```python
from build123d import *

# Parameters (mm, degrees)
F0_W     = 31.6992
F0_H     = 15.9004
F0_R     = 2.3876
F1_DEPTH = 3.175
F2_DEPTH = 4.7752
F3_T     = -1.6002


with BuildPart() as f1:
    # F0 (on Top) → F1 (new body)
    with BuildSketch(Plane.XY):
        with Locations((0.5139857531, -7.2151332219)):
            Rectangle(F0_W, F0_H)
        with Locations((-11.3732142469, -11.1521332219)):
            Circle(F0_R, mode=Mode.SUBTRACT)
        with Locations((-3.4230142469, -11.1521332219)):
            Circle(F0_R, mode=Mode.SUBTRACT)
        with Locations((4.5271857531, -11.1521332219)):
            Circle(F0_R, mode=Mode.SUBTRACT)
        with Locations((12.4773857531, -11.1521332219)):
            Circle(F0_R, mode=Mode.SUBTRACT)
        with Locations((-11.3732142469, -3.2273332219)):
            Circle(F0_R, mode=Mode.SUBTRACT)
        with Locations((-3.4230142469, -3.2273332219)):
            Circle(F0_R, mode=Mode.SUBTRACT)
        with Locations((4.5271857531, -3.2273332219)):
            Circle(F0_R, mode=Mode.SUBTRACT)
        with Locations((12.4773857531, -3.2273332219)):
            Circle(F0_R, mode=Mode.SUBTRACT)
    extrude(amount=F1_DEPTH)

    # F0 (on Top) → F2 (join)
    with BuildSketch(Plane.XY):
        with Locations((-11.3732142469, -3.2273332219)):
            Circle(F0_R)
        with Locations((-3.4230142469, -3.2273332219)):
            Circle(F0_R)
        with Locations((4.5271857531, -3.2273332219)):
            Circle(F0_R)
        with Locations((12.4773857531, -3.2273332219)):
            Circle(F0_R)
        with Locations((12.4773857531, -11.1521332219)):
            Circle(F0_R)
        with Locations((4.5271857531, -11.1521332219)):
            Circle(F0_R)
        with Locations((-3.4230142469, -11.1521332219)):
            Circle(F0_R)
        with Locations((-11.3732142469, -11.1521332219)):
            Circle(F0_R)
    extrude(amount=F2_DEPTH)

    # F3
    f3_openings = [f1.faces().sort_by_distance(p)[0] for p in [
        (0.513986, -7.215133, 0),
    ]]
    offset(amount=F3_T, openings=f3_openings, kind=Kind.INTERSECTION)


solid = f1.part
```
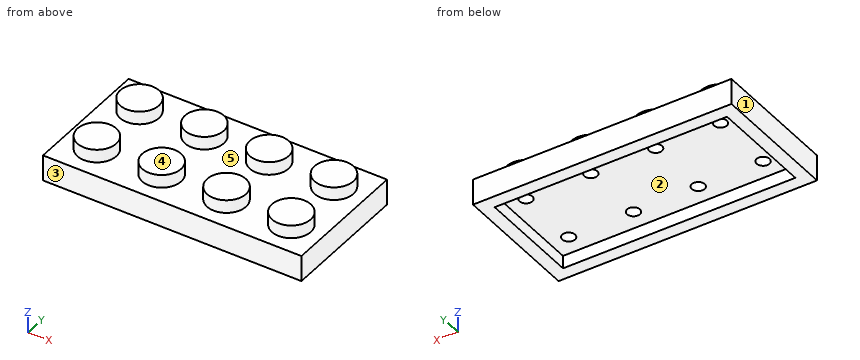
Input: part model. Units: mm. Frame: model coordinates. Face numbers are marked on the shaded views. A direction names the side the tool comes from. Round coordinates to 2 decimals unless told otherwise and drop trailing zeros. Loops run counter-clockwise (first coordinate to the right, second up) from the corner with the lowest first, then second, coordinate; pieces in that order, holes last. Notation, with made-up numbers: (-19, 60) -> (19, 60) arc R18 ccw to (19, 71) -> close; hole circle Ø7 at (18.25, 35). An arc over 180 degrees is marked (long way). Use one line per item in the form item = value. Start each with the question number.
Item 1: Material intervals for L1, parallel to Y at x = 14, z = 0.45; L2, parallel to X at y = -12.5, z = 0.3; L3, parallel to X at y = -3.5, z = 4.15 (3 decimals), sorted ascending. Write a range as from..to.
Item 2: Mould query, pull axis Y, two halves, no side actions, for the marked faces 1, 2 and 3. Classes: pulls with the +Y half, pulls with the -Y half, needs draft (parallel to the pull), parting line crosses it, or undercut.
Item 3: Section query D-D on z = 3.5. Return the cut outline in (x, y), then the cut area to 3 significant figures.
Item 4: Section query C-C on x = -3.5. Return the cut outline in (y, z) (1 decimal), then the cut area to 3 significant figures.
Item 5: Set-up query: the marked faces 4 and 5. Return all of +Z, -Z, +X, -X, +Y, -Y with unobstructed straight access to the full face (end or side cutting, diameter ignored); none if empty.
Item 6: Section query B-B on y = -7.75. Return the cut outline in (x, z) (3 decimals).
Item 7: Section query A-A on z = 1.05. Return the cut outline in (x, y).
Item 8: Contact query for flat-ended pins moving along their axis: pin 1 Ø1.3 at (x, y) = (-3.5, -3.5) entering from -Z; pin 2 Ø1 at (x, z) = (-6, 3.5) entering from +Y; pin 3 Ø1.4 at (x, y) = (-11.37, -11.15) entering from -Z (3 decimals). Output: stop coordinate, or through.
Ans:
q1.L1 = -15.17..-13.57, -0.87..0.74
q1.L2 = -15.34..-13.74, 14.76..16.36
q1.L3 = -13.745..-9.001, -5.795..-1.051, 2.155..6.899, 10.105..14.849
q2.face_1 = needs draft
q2.face_2 = undercut
q2.face_3 = pulls with the -Y half
q3.outline = circle Ø4.78 at (-11.37, -11.15); circle Ø4.78 at (-11.37, -3.23); circle Ø4.78 at (-3.42, -11.15); circle Ø4.78 at (-3.42, -3.23); circle Ø4.78 at (4.53, -11.15); circle Ø4.78 at (4.53, -3.23); circle Ø4.78 at (12.48, -11.15); circle Ø4.78 at (12.48, -3.23)
q3.area = 143 mm^2
q4.outline = (-15.2, 0) -> (-13.6, 0) -> (-13.6, 1.6) -> (-11.9, 1.6) -> (-11.9, 3.2) -> (-10.4, 3.2) -> (-10.4, 1.6) -> (-4, 1.6) -> (-4, 3.2) -> (-2.4, 3.2) -> (-2.4, 1.6) -> (-0.9, 1.6) -> (-0.9, 0) -> (0.7, 0) -> (0.7, 3.2) -> (-0.8, 3.2) -> (-0.8, 4.8) -> (-5.6, 4.8) -> (-5.6, 3.2) -> (-8.8, 3.2) -> (-8.8, 4.8) -> (-13.5, 4.8) -> (-13.5, 3.2) -> (-15.2, 3.2) -> close
q4.area = 40.7 mm^2
q5.face_4 = +Z, +X, -X, +Y, -Y
q5.face_5 = +Z
q6.outline = (-15.336, 0) -> (-13.735, 0) -> (-13.735, 1.575) -> (14.763, 1.575) -> (14.763, 0) -> (16.364, 0) -> (16.364, 3.175) -> (-15.336, 3.175) -> close
q7.outline = (-15.34, -15.17) -> (16.36, -15.17) -> (16.36, 0.74) -> (-15.34, 0.74) -> close; hole (-13.74, -13.57) -> (14.76, -13.57) -> (14.76, -0.87) -> (-13.74, -0.87) -> close
q8.pin_1 = 1.57
q8.pin_2 = 0.74
q8.pin_3 = 3.175
